from build123d import *

# Parameters (mm, degrees)
F2_R     = 3.175
F3_DEPTH = 25.4


# Not quite as in the source:
# - a feature names something its author has since deleted; it is built from what else it names


with BuildPart() as f3:
    # F2 (on Front) → F3 (new body)
    with BuildSketch(Plane.XZ):
        with BuildLine():
            ThreePointArc((15.7504884308, 65.4843737526), (6.286e-07, 79.375), (-15.7504882737, 65.484375))
            ThreePointArc((-15.7504882737, 65.484375), (-15.8738192656, 63.6936154008), (-15.7942028036, 61.9003804205))
            ThreePointArc((-15.7942028036, 61.9003804205), (0.0060905531, 47.6250011683), (15.7954255641, 61.9125))
            ThreePointArc((15.7954255641, 61.9125), (15.8550939106, 62.7052534459), (15.875, 63.5))
            ThreePointArc((15.875, 63.5), (15.8438415297, 64.4941381092), (15.7504884308, 65.4843737526))
        make_face()
        with Locations((0, 63.5)):
            Circle(F2_R, mode=Mode.SUBTRACT)
        with BuildLine():
            Line((-9.4502929642, 115.490625), (-15.7504882737, 65.484375))
            ThreePointArc((-15.7504882737, 65.484375), (6.286e-07, 79.375), (15.7504884308, 65.4843737526))
            Line((15.7504884308, 65.4843737526), (9.4502929642, 115.490625))
            ThreePointArc((9.4502929642, 115.490625), (9.5063048942, 114.896483242), (9.525, 114.3))
            ThreePointArc((9.525, 114.3), (-0.596483242, 104.7936951058), (-9.4502929642, 115.490625))
        make_face()
        with Locations((-3.175, 100.0252)):
            Circle(F2_R, mode=Mode.SUBTRACT)
        with BuildLine():
            ThreePointArc((15.7954255641, 61.9125), (0.0060905531, 47.6250011683), (-15.7942028036, 61.9003804205))
            Line((-15.7942028036, 61.9003804205), (-9.525, 0))
            ThreePointArc((-9.525, 0), (0, 9.525), (9.525, 0))
            ThreePointArc((9.525, 0), (6.9705567315, -6.4912990883), (0.6773435479, -9.500885786))
            Line((0.6773435479, -9.500885786), (44.7324052746, -7.9324746146))
            ThreePointArc((44.7324052746, -7.9324746146), (36.5125, 0), (44.7324052746, 7.9324746146))
            Line((44.7324052746, 7.9324746146), (18.968327868, 8.8497055806))
            ThreePointArc((18.968327868, 8.8497055806), (13.2612039825, 11.5674628959), (11.3408358685, 17.5898921545))
            Line((11.3408358685, 17.5898921545), (15.7954255641, 61.9125))
        make_face()
        with BuildLine():
            ThreePointArc((9.4502929642, 115.490625), (0, 123.825), (-9.4502929642, 115.490625))
            ThreePointArc((-9.4502929642, 115.490625), (-0.596483242, 104.7936951058), (9.525, 114.3))
            ThreePointArc((9.525, 114.3), (9.5063048942, 114.896483242), (9.4502929642, 115.490625))
        make_face()
        with Locations((0, 114.3)):
            Circle(F2_R, mode=Mode.SUBTRACT)
        with BuildLine():
            ThreePointArc((9.525, 0), (0, 9.525), (-9.525, 0))
            ThreePointArc((-9.525, 0), (-6.7351920908, -6.7351920908), (0, -9.525))
            Line((0, -9.525), (0.6773435479, -9.500885786))
            ThreePointArc((0.6773435479, -9.500885786), (6.9705567315, -6.4912990883), (9.525, 0))
        make_face()
        Circle(F2_R, mode=Mode.SUBTRACT)
        with BuildLine():
            Line((0.6773435479, -9.500885786), (0, -9.525))
            ThreePointArc((0, -9.525), (0.3388863295, -9.5189695375), (0.6773435479, -9.500885786))
        make_face()
        with BuildLine():
            ThreePointArc((52.3875, 0), (50.1616327839, 5.5119104847), (44.7324052746, 7.9324746146))
            ThreePointArc((44.7324052746, 7.9324746146), (36.5125, 0), (44.7324052746, -7.9324746146))
            ThreePointArc((44.7324052746, -7.9324746146), (50.1616327839, -5.5119104847), (52.3875, 0))
        make_face()
        with Locations((44.45, 0)):
            Circle(F2_R, mode=Mode.SUBTRACT)
    extrude(amount=F3_DEPTH)


solid = f3.part
Could you check a few things on this model? Use its own coordinates, in mm. A direction names the side the tool comes from. Coordinates: 2 decimals unless noted, no trailing zeros. Order: outer loops, then holes, each group sorted by start corner. A loop starts at its lowest first (then second) coordinate and runs counter-clockwise, first axis right, second up. Notation, with made-up numbers: (41, 2.5) - (75, 2.5) arc R18 ccw to (75, 36.5) - close; hole circle Ø11 at (45, -10.75). An arc over 180 degrees is marked (long way). Answer in a Markdown table with one row per item. Add a question column.
(1) If we section it at B-B, the plane y = -3.75: State how many separate pieces and enclosed holes the cut face has, then the cut area to 3 significant figures.
(2) If we section it at C-C, the plane z = 104.5: Please give me the cut outline in (x, y), then the cut area to 3 significant figures.
(3) I need wall thicknesses on L1, parallel to Z at x = 44.45, y = -18.5 (3 decimals); L2, parallel to X at y = -1.5, z = 98.5; L3, parallel to X at y = -18.5, z = 16. Which ranges of each line are inside material? Lowest first, please.
(4) Will these pins go through, and if not, where does the flat tip stop? pin 1 (2 mm diameter, centred on y = -5, z = 87.5, fed in from +X); pin 2 (1 mm diameter, centred on x = -1, y = -13.5, fed in from -Z); pin 3 (1 mm diameter, centred on x = 28.5, y = -19.5, fed in from +Z); pin 4 (10 mm diameter, centred on x = 0, z = 114.3, fed in from -Y).
(5) If we mould it in two halves opening along X, with no side actions, what happens to faces 3 (the face through (1.707, -12.522, 66.177)), 4 (the face through (3, 0, 43)), 5 (the face through (0.193, -12.522, 123.823))? For each: released by +X, released by -X, zero draft, split by the parting line, or undercut.
(6) If we section it at D-D, the plane x = 26.5: Please give me the cut outline in (y, z), then the cut area to 3 significant figures.
(7) If we section it at A-A, the plane x = -5: Please give me the cut outline in (y, z), then the cut area to 3 significant figures.
(8) On a 3-axis mill with a long thin cutter (end or side, diameter ignored), from which of +Z, -Z, +X, -X, +Y, -Y can I reach the whole of each face in a straight line? I mean faces 1 (the face through (-12.556, -12.522, 90.838)), 2 (the face through (13.32, -12.52, 11.5)). Say none if no direction works.
Results are:
| question | item | result |
|---|---|---|
| 1 | separate pieces | 1 |
| 1 | enclosed holes | 5 |
| 1 | area | 3,770 mm2 |
| 2 | outline | (-10.83, -25.4) - (10.83, -25.4) - (10.83, 0) - (-10.83, 0) - close |
| 2 | area | 550 mm2 |
| 3 | L1 | z = -7.943 to -3.175, 3.175 to 7.943 |
| 3 | L2 | x = -11.59 to -5.96, -0.39 to 11.59 |
| 3 | L3 | x = -11.15 to 11.34 |
| 4 | pin 1 | stops at x = 13.1 |
| 4 | pin 2 | stops at z = -9.51 |
| 4 | pin 3 | stops at z = 8.53 |
| 4 | pin 4 | stops at y = -25.4 |
| 5 | face 3 | undercut |
| 5 | face 4 | zero draft |
| 5 | face 5 | split by the parting line |
| 6 | outline | (-25.4, -8.58) - (0, -8.58) - (0, 8.58) - (-25.4, 8.58) - close |
| 6 | area | 436 mm2 |
| 7 | outline | (-25.4, -8.11) - (0, -8.11) - (0, 97.43) - (-25.4, 97.43) - close; (-25.4, 102.62) - (0, 102.62) - (0, 122.41) - (-25.4, 122.41) - close |
| 7 | area | 3,180 mm2 |
| 8 | face 1 | +Z, -X, +Y, -Y |
| 8 | face 2 | +X, +Y, -Y |
